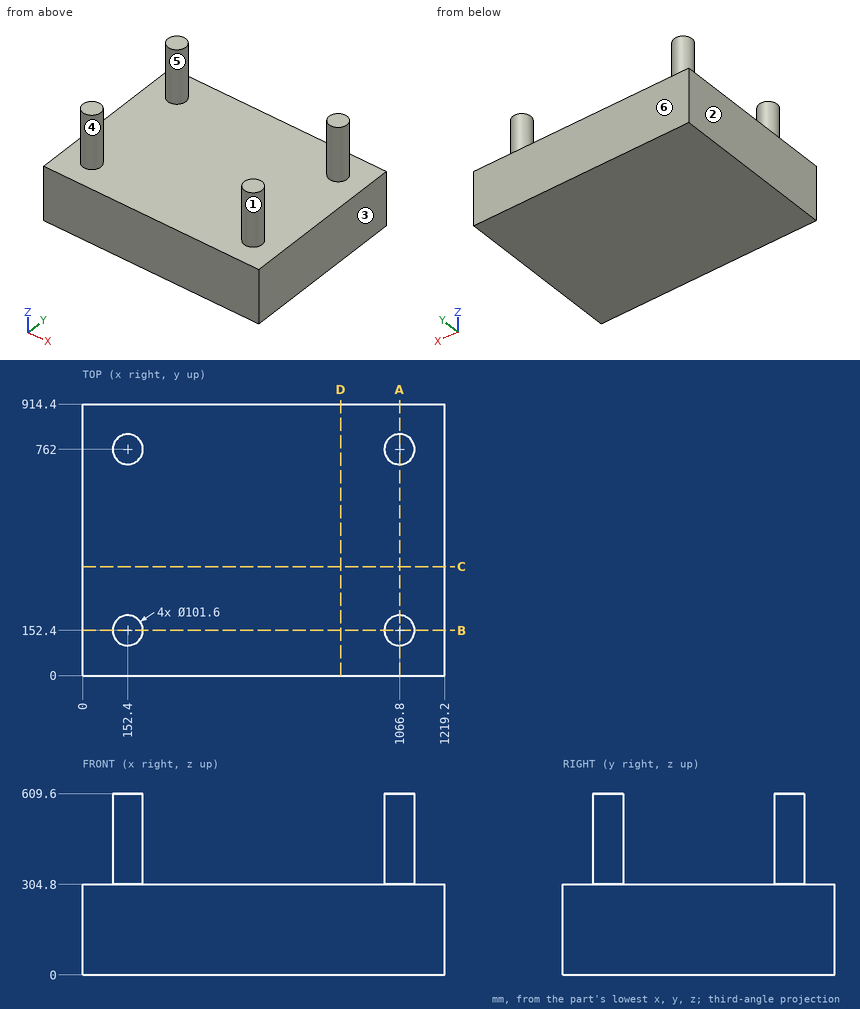
Answer from the drawing. Dimensions are ordinates in mm from the lowest x, y and z of the part. A direction names the side the tool comes from. Give positions to 0.01 mm unless a question says otherwise; leave off trailing zeros. Order: outer loops, then holes, each group sorted by start corner. A loop starts at its lowest first (then second) coordinate and runs counter-clockwise, first axis right, second up. Notation, with made-up numbers: (61.5, -13) -> (78.5, -13) arc R19 ccw to (78.5, -7) -> close; hole circle Ø6 at (73.25, 8.5). An arc over 180 degrees is marked (long way). One line per item, written item: value. Start each with the question number.
(1) Straight lines are drawn through the part: L1, parallel to Z at x = 729.5, y = 247.5; L2, parallel to X at y = 741.5, z = 490; L3, parallel to Y at x = 1044.5, z = 436. For each, find the intervals that lie inside material, in ascending order.
(2) A flat-ended cylindrical pin translates along its axis: P1, Ø2, axis at y = 788.5, z = 311.5, coming from the -X side. Find the tip coordinate at first contact, or state that the pin passes through.
(3) The part is cut by section B-B (y = 152.4). Determine the outline of the cut face in (x, z), and give its area (3 significant figures).
(4) The part is cut by section A-A (x = 1066.8). Determine the outline of the cut face in (y, z), and give its area (3 significant figures).
(5) For a pull along X with two mould halves and no side action, classify the marked faces 3, 4, 5 and 6 as released by +X, released by -X, zero draft, split by the parting line, or undercut.
(6) A tool of negligible diameter and unlimited length cuts with its end or side. For the marked faces 1 and 2, from which of +Z, -Z, +X, -X, +Y, -Y can it reach the whole face along a straight path? Write none if from no direction.
(7) The part is cut by section C-C (y = 367.5). Determine the outline of the cut face in (x, z).
(8) The part is cut by section D-D (x = 868.5). Determine the outline of the cut face in (y, z), and give its area (3 significant figures).
Taken from the geometry:
1. L1: 0 to 304.8
1. L2: 105.92 to 198.88, 1020.32 to 1113.28
1. L3: 106.76 to 198.04, 716.36 to 807.64
2. P1: x = 108.46
3. outline: (0, 0) -> (1219.2, 0) -> (1219.2, 304.8) -> (1117.6, 304.8) -> (1117.6, 609.6) -> (1016, 609.6) -> (1016, 304.8) -> (203.2, 304.8) -> (203.2, 609.6) -> (101.6, 609.6) -> (101.6, 304.8) -> (0, 304.8) -> close
3. area: 434,000 mm^2
4. outline: (0, 0) -> (914.4, 0) -> (914.4, 304.8) -> (812.8, 304.8) -> (812.8, 609.6) -> (711.2, 609.6) -> (711.2, 304.8) -> (203.2, 304.8) -> (203.2, 609.6) -> (101.6, 609.6) -> (101.6, 304.8) -> (0, 304.8) -> close
4. area: 341,000 mm^2
5. face 3: released by +X
5. face 4: undercut
5. face 5: undercut
5. face 6: zero draft
6. face 1: +Z
6. face 2: +Z, -Z, -X, +Y, -Y
7. outline: (0, 0) -> (1219.2, 0) -> (1219.2, 304.8) -> (0, 304.8) -> close
8. outline: (0, 0) -> (914.4, 0) -> (914.4, 304.8) -> (0, 304.8) -> close
8. area: 279,000 mm^2
